Could you check a few things on this model? Use its own coordinates, in mm. A direction names the side the tool comes from. Round coordinates to 2 decimals unless told otherwise and drop trailing zeros. Loops run counter-clockwise (first coordinate to the right, second up) from the corner with the lowest first, then second, coordinate; pieces in that order, holes last. Notation, with made-up numbers: (81.5, 75) -> (101.5, 75) arc R26 ccw to (101.5, 91) -> close; hole circle Ø7 at (3, -0.75). An arc over 180 degrees is marked (long way). One line per item, written item: value.
from build123d import *

# Parameters (mm, degrees)
BOSS_EXTRUDE1_DEPTH     = 70
BOSS_EXTRUDE2_DEPTH     = 60
SKETCH4_W               = 40
SKETCH4_H               = 20
CUT_EXTRUDE1_DEPTH      = 41
CUT_EXTRUDE1_DEPTH_BACK = 41


with BuildPart() as part:
    # Sketch1 → Boss-Extrude1 (new body)
    with BuildSketch(Plane(origin=(0, 0, 0), x_dir=(1, 0, 0), z_dir=(0, 1, 0))):
        with BuildLine():
            ThreePointArc((40, 0), (28.284271247, 28.284271247), (0, 40))
            Line((0, 40), (0, 25))
            ThreePointArc((0, 25), (17.67766953, 17.67766953), (25, 0))
            ThreePointArc((25, 0), (17.67766953, -17.67766953), (0, -25))
            Line((0, -25), (0, -40))
            ThreePointArc((0, -40), (28.284271247, -28.284271247), (40, 0))
        make_face()
        with BuildLine():
            Line((0, -40), (0, -25))
            ThreePointArc((0, -25), (-13.693063938, -20.916500663), (-22.912878475, -10))
            Line((-22.912878475, -10), (-38.729833462, -10))
            ThreePointArc((-38.729833462, -10), (-24.494897428, -31.622776602), (0, -40))
        make_face()
        with BuildLine():
            Line((0, 25), (0, 40))
            ThreePointArc((0, 40), (-24.494897428, 31.622776602), (-38.729833462, 10))
            Line((-38.729833462, 10), (-22.912878475, 10))
            ThreePointArc((-22.912878475, 10), (-13.693063938, 20.916500663), (0, 25))
        make_face()
    extrude(amount=BOSS_EXTRUDE1_DEPTH)

    # Sketch1_3 → Boss-Extrude2 (add)
    with BuildSketch(Plane(origin=(0, 0, 0), x_dir=(1, 0, 0), z_dir=(0, 1, 0))):
        with BuildLine():
            Line((-22.912878475, 10), (-38.729833462, 10))
            ThreePointArc((-38.729833462, 10), (-40, 0), (-38.729833462, -10))
            Line((-38.729833462, -10), (-22.912878475, -10))
            ThreePointArc((-22.912878475, -10), (-25, 0), (-22.912878475, 10))
        make_face()
    extrude(amount=BOSS_EXTRUDE2_DEPTH)

    # Sketch4 → Cut-Extrude1 (cut, two sides)
    with BuildSketch(Plane.XY) as cut_extrude1_sk:
        Polygon((40, 50), (0, 50), (40, 20), align=None)
        with Locations((20, 60)):
            Rectangle(SKETCH4_W, SKETCH4_H)
    extrude(amount=CUT_EXTRUDE1_DEPTH, mode=Mode.SUBTRACT)
    extrude(cut_extrude1_sk.sketch, amount=-CUT_EXTRUDE1_DEPTH_BACK, mode=Mode.SUBTRACT)


solid = part.part
(1) I'm going to push flat-ended pins straight in: pin 1 Ø7.5 at (y, z) = (61.5, -30) entering from +X; pin 2 Ø1.5 at (y, z) = (56, -6.5) entering from -X; pin 3 Ø8.5 at (x, z) = (-31.5, 3) entering from +Y. Where does each tip first touch, or does it pass through?
Recorded:
pin 1: x = 0
pin 2: x = -39.58
pin 3: y = 60
(2) Thinking about a two-plate mould opening in Z: for faces 4 (the face through (-32, 60, 0)), 5 (the face through (-20, 70, -25)), which applies, released by +Z, released by -Z, zero draft, split by the parting line, or undercut?
Recorded:
face 4: undercut
face 5: zero draft
(3) For faces 1 (the face through (0, 60, -32)), 2 (the face through (-31, 65, -10)), 3 (the face through (17.22, 0, -18.34)), which set-ups out of +Z, -Z, +X, -X, +Y, -Y let a thin tool reach every point of the face, with its end or its side?
Recorded:
face 1: +Z, -Z, +X, +Y
face 2: +X, -X, +Y
face 3: +Z, -Z, +X, -X, -Y
(4) If I drill on L1, parallel to X at y = 29.5, z = -22.5; L2, parallel to Z at x = -12, y = 19; L3, parallel to Z at x = -31.5, y = 61, over which ranges is the centre line in solid material (lowest first)?
Recorded:
L1: -33.07 to -10.9, 10.9 to 27.33
L2: -38.16 to -21.93, 21.93 to 38.16
L3: -24.65 to -10, 10 to 24.65
(5) If we section it at B-B, the plane x = 6: Please give me the cut outline in (y, z), then the cut area to 3 significant figures.
Recorded:
outline: (0, -39.55) -> (45.5, -39.55) -> (45.5, -24.27) -> (0, -24.27) -> close; (0, 24.27) -> (45.5, 24.27) -> (45.5, 39.55) -> (0, 39.55) -> close
area: 1,390 mm²
(6) If we section it at C-C, the plane z = 16: Please give me the cut outline in (x, y), then the cut area to 3 significant figures.
Recorded:
outline: (-36.66, 0) -> (-19.21, 0) -> (-19.21, 70) -> (-36.66, 70) -> close; (19.21, 0) -> (36.66, 0) -> (36.66, 22.5) -> (19.21, 35.59) -> close
area: 1,730 mm²
(7) If we section it at D-D, the plane y = 56.5: Please give me the cut outline in (x, z), then the cut area to 3 significant figures.
Recorded:
outline: (0, -40) -> (0, -25) arc R25 cw to (0, 25) -> (0, 40) arc R40 ccw to start
area: 1,530 mm²
(8) If we section it at A-A, the plane y = 8: Please give me the cut outline in (x, z), then the cut area to 3 significant figures.
Recorded:
outline: circle Ø80 at (0, 0); hole circle Ø50 at (0, 0)
area: 3,060 mm²
